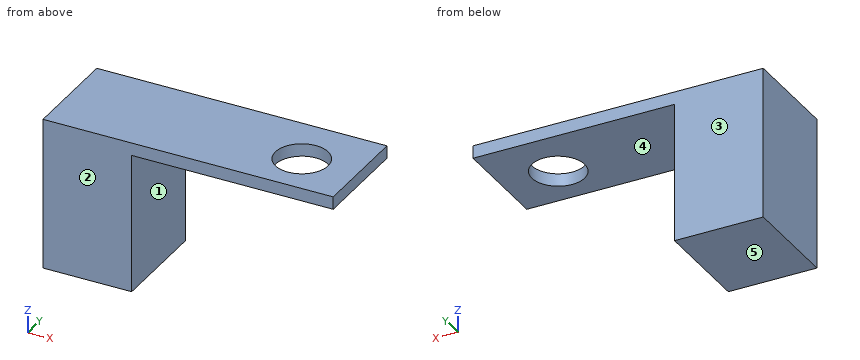
```python
from build123d import *

# Parameters (mm, degrees)
F0_W     = 533.4
F0_H     = 914.4
F1_DEPTH = 609.6
F2_W     = 1211.786538
F2_H     = 609.6
F3_DEPTH = 76.2
F4_R     = 158.514697
F5_DEPTH = 914.401


with BuildPart() as f1:
    # F0 (on Front) → F1 (new body)
    with BuildSketch(Plane.XZ):
        Rectangle(F0_W, F0_H)
    extrude(amount=-F1_DEPTH)

    # F2 (on face) → F3 (join)
    with BuildSketch(Plane.XY.offset(457.2)):
        with Locations((872.593269, 304.8)):
            Rectangle(F2_W, F2_H)
    extrude(amount=-F3_DEPTH)

    # F4 (on face) → F5 (cut, through all)
    with BuildSketch(Plane.XY.offset(457.2)):
        with Locations((1142.773271, 276.569486)):
            Circle(F4_R)
    extrude(amount=-F5_DEPTH, mode=Mode.SUBTRACT)


solid = f1.part
```
Model file for the job. Use its own axes, mm. Face numbers are marked on the shaded views. A direction names the side the tool comes from. Coordinates: 2 decimals unless noted, no trailing zeros. Order: outer loops, then holes, each group sorted by start corner. A loop starts at its lowest first (then second) coordinate and runs counter-clockwise, first axis right, second up. Notation, with made-up numbers: (23.25, -34.5) - (75.25, -34.5) arc R30 ccw to (75.25, -4.5) - close; hole circle Ø6 at (60, 5). An arc over 180 degrees is marked (long way). Return JSON: item names as keys, results as strings. Group by question number.
1) Mould opens along Y. For the marked faces 1, 2 and 3 say: released by +Y, released by -Y, zero draft, split by the parting line, or undercut.
2) Saw through at D-D, the plane x = 566.5. Write the cut outline in (y, z), plus the area to 3 significant figures.
3) Saw through at B-B, the plane y = 218. Write the cut outline in (x, z), plus the area to 3 significant figures.
4) Probe line 1 (Z direction, x = 754, y = 262); line 2 (X direction, y = 137.5, z = 73). List the from-to ranges inside material, lowest first. Write a range as from..to.
5) Tool access for the marked faces 4 and 5: list every direction of +Z, -Z, +X, -X, +Y, -Y with a clear straight run to the whole face (end or side of a thin tool).
6) Saw through at C-C, the plane y = 536.5. Write the cut outline in (x, z), plus the area to 3 significant figures.
7) Flat gauge pins, fed straight in: P1, Ø1, axis at x = 12, z = -285.5, coming from the -Y side; P2, Ø1, axis at y = 325, z = -181, coming from the +X side; P3, Ø5, axis at x = 600.5, y = 503.5, coming from the -Z side. Where does each tip first touch, or does it go through?
8) Saw through at A-A, the plane x = 1119.5. Write the cut outline in (y, z), plus the area to 3 significant figures.
Values found:
{
 "1": {"face 1": "zero draft", "face 2": "released by -Y", "face 3": "released by +Y"},
 "2": {"outline": "(0, 381) - (609.6, 381) - (609.6, 457.2) - (0, 457.2) - close", "area": "46,500 mm²"},
 "3": {"outline": "(-266.7, -457.2) - (266.7, -457.2) - (266.7, 381) - (995.48, 381) - (995.48, 457.2) - (-266.7, 457.2) - close; (1290.07, 381) - (1478.49, 381) - (1478.49, 457.2) - (1290.07, 457.2) - close", "area": "558,000 mm²"},
 "4": {"line 1": "z = 381..457.2", "line 2": "x = -266.7..266.7"},
 "5": {"face 4": "-Z, +X, +Y, -Y", "face 5": "-Z, +X, -X, +Y, -Y"},
 "6": {"outline": "(-266.7, -457.2) - (266.7, -457.2) - (266.7, 381) - (1478.49, 381) - (1478.49, 457.2) - (-266.7, 457.2) - close", "area": "580,000 mm²"},
 "7": {"P1": "stops at y = 0", "P2": "stops at x = 266.7", "P3": "stops at z = 381"},
 "8": {"outline": "(0, 381) - (119.77, 381) - (119.77, 457.2) - (0, 457.2) - close; (433.37, 381) - (609.6, 381) - (609.6, 457.2) - (433.37, 457.2) - close", "area": "22,600 mm²"}
}
